Geometry check sheet. Reference: the model listing, model coordinates, mm. Face numbers are marked on the shaded views. A direction names the side the tool comes from. Coordinates: 2 decimals unless noted, no trailing zeros. Loops run counter-clockwise (first coordinate to the right, second up) from the corner with the lowest first, then second, coordinate; pieces in that order, holes last.
from build123d import *

# Parameters (mm, degrees)
F0_W     = 15
F0_H     = 20
F1_DEPTH = 5
F2_W     = 2.8
F2_H     = 5
F3_DEPTH = 3
F4_W     = 2.8
F4_H     = 2.5
F6_R     = 1.4
F7_DEPTH = 5


with BuildPart() as f1:
    # F0 (on Top) → F1 (new body)
    with BuildSketch(Plane.XY):
        Rectangle(F0_W, F0_H)
    extrude(amount=F1_DEPTH)

    # F2 (on face) → F3 (join)
    with BuildSketch(Plane.XZ.offset(10)):
        with Locations((0, 2.5)):
            Rectangle(F2_W, F2_H)
    extrude(amount=F3_DEPTH)

    # F4 (on face) → F5 (revolve)
    with BuildSketch(Plane.XZ.offset(13)):
        with Locations((0, 1.25)):
            Rectangle(F4_W, F4_H)
    revolve(axis=Axis((0, -13, 2.5), (1, 0, 0)))

    # F6 (on face) → F7 (cut)
    with BuildSketch(Plane(origin=(-1.4, 0, 0), x_dir=(0, -1, 0), z_dir=(-1, 0, 0))):
        with Locations((13, 2.5)):
            Circle(F6_R)
    extrude(amount=-F7_DEPTH, mode=Mode.SUBTRACT)


solid = f1.part
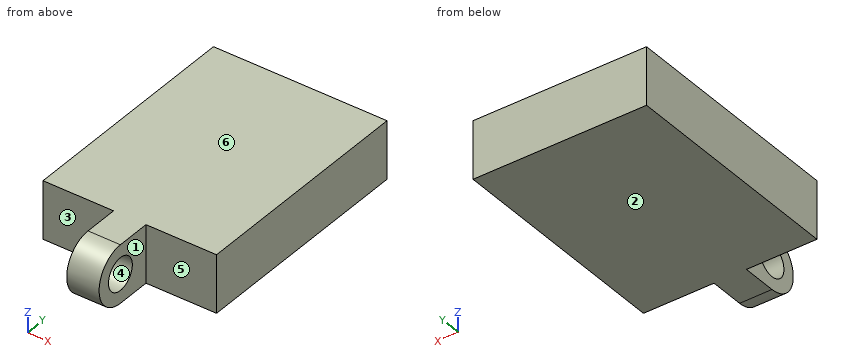
1) Section check A-A on z = 2.5. Record the cut outline in (x, y).
Data:
outline: (-7.5, -10) - (-1.4, -10) - (-1.4, -11.6) - (1.4, -11.6) - (1.4, -10) - (7.5, -10) - (7.5, 10) - (-7.5, 10) - close; (-1.4, -15.5) - (1.4, -15.5) - (1.4, -14.4) - (-1.4, -14.4) - close
2) Mould release check, pull along Z, two halves, no side actions. Record for the marked faces 4, 5 and 6: +Z half, -Z half, draft (parallel to the pull), parting line (faces both ways), or undercut.
Data:
face 4: undercut
face 5: draft
face 6: +Z half
3) Depth check by flat-ended pin: pin 1 (1.5 mm diameter, centred on y = -13.5, z = 2.5, fed in from +X); pin 2 (1 mm diameter, centred on x = -2.5, z = 2, fed in from -Y); pin 3 (1.5 mm diameter, centred on y = -12.5, z = 1.5, fed in from -X). Enter the tip coordinate at first touch or a pass-through.
Data:
pin 1: passes through
pin 2: stops at y = -10
pin 3: stops at x = -1.4
4) Section check C-C on z = 4.2. Record the cut outline in (x, y).
Data:
outline: (-7.5, -10) - (-1.4, -10) - (-1.4, -14.83) - (1.4, -14.83) - (1.4, -10) - (7.5, -10) - (7.5, 10) - (-7.5, 10) - close
5) Access from +Z, -Z, +X, -X, +Y, -Y to the whole of each face (thin tool, end or side, straight path). Record for the marked faces 1, 2 and 3.
Data:
face 1: +Z, -Z, +X, -Y
face 2: -Z, +X, -X, +Y, -Y
face 3: +Z, -Z, -X, -Y
6) Material ranges on probe 1 along Z at (x, y) = (-0.8, -13); probe 2 along Y at (x, z) = (6.75, 3.65); probe 3 along X at (y, z) = (-11.25, 2.2), recorded low to high.
Data:
probe 1: z = 0 to 1.1, 3.9 to 5
probe 2: y = -10 to 10
probe 3: x = -1.4 to 1.4
7) Section check D-D on z = 0.45. Record the cut outline in (x, y), and give its area (3 significant figures).
Data:
outline: (-7.5, -10) - (-1.4, -10) - (-1.4, -14.43) - (1.4, -14.43) - (1.4, -10) - (7.5, -10) - (7.5, 10) - (-7.5, 10) - close
area: 312 mm2
8) Section check B-B on x = 3.75. Record the cut outline in (y, z), and give its area (3 significant figures).
Data:
outline: (-10, 0) - (10, 0) - (10, 5) - (-10, 5) - close
area: 100 mm2
